Source: three-view drawing plus pictorial views. Frame: mm from the lowest corner of the part. A direction names the side the tool comes from. Give positions to 0.01 mm unless a question says otherwise; leave off trailing zeros. Loops run counter-clockwise (first coordinate to the right, second up) from the corner with the lowest first, then second, coordinate; pieces in that order, holes last. Notation, with made-up numbers: (78.25, -18.75) - (82.25, -18.75) arc R32 ccw to (82.25, 19.25) - close; hole circle Ø6 at (-17.75, -7.5). An arc over 180 degrees is marked (long way). One line per item, written item: value.
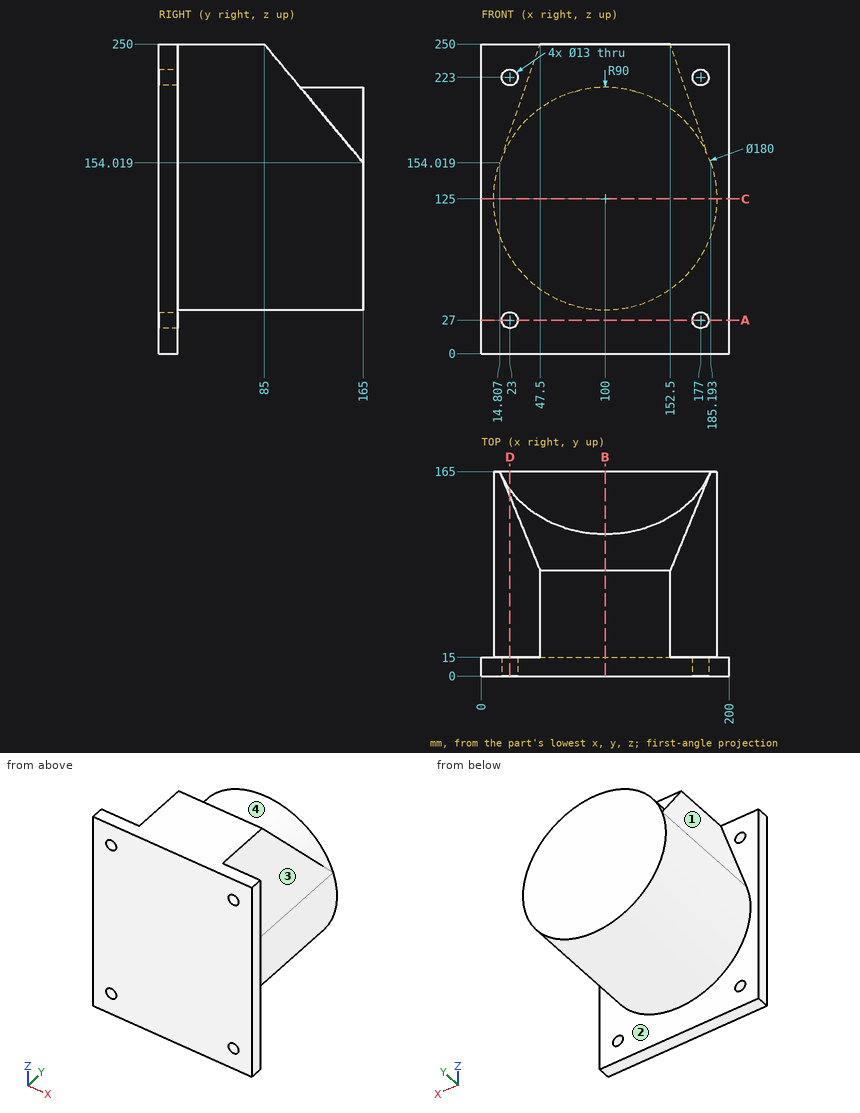
Item 1: Pin query (flat end, axial travel): P1, Ø3, axis at y = 24, z = 124, coming from the -X side; P2, Ø1, axis at y = 131.5, z = 206, coming from the +X side (1 decimal); P3, Ø2, axis at x = 113.5, y = 42, coming from the -Z side. Return the tip coordinate at first contact, or that it passes through.
Verdict:
P1: stops at x = 10
P2: stops at x = 140.2
P3: stops at z = 35.87
Item 2: Section A-A, the plane z = 27. Output: boundary loops of the cut face in (x, y).
Verdict:
outline: (0, 0) - (16.5, 0) - (16.5, 15) - (0, 15) - close; (29.5, 0) - (170.5, 0) - (170.5, 15) - (29.5, 15) - close; (183.5, 0) - (200, 0) - (200, 15) - (183.5, 15) - close
Item 3: Material intervals for L1, parallel to X at y = 9, z = 223; L2, parallel to Y at x = 184, z = 222; L3, parallel to Z at x = 139.5, y = 20.5, sorted ascending.
Verdict:
L1: x = 0 to 16.5, 29.5 to 170.5, 183.5 to 200
L2: y = 0 to 15
L3: z = 44.13 to 250
Item 4: Access query for the marked faces 1, 2, 3 and 4. Directions: +Z, -Z, +X, -X, +Y, -Y. A direction counts if a zero-diameter tool reaches every point of the face in a straight line with its end or side. Return the directions, or none.
Verdict:
face 1: +Z, -X, +Y
face 2: +Y
face 3: +Z, +X, +Y
face 4: +Z, +Y
Item 5: Section C-C, the plane z = 125. Output: boundary loops of the cut face in (x, y).
Verdict:
outline: (0, 0) - (200, 0) - (200, 15) - (190, 15) - (190, 165) - (10, 165) - (10, 15) - (0, 15) - close
Item 6: Section B-B, the plane x = 100. Output: boundary loops of the cut face in (y, z), and give its area (3 significant figures).
Verdict:
outline: (0, 0) - (15, 0) - (15, 35) - (165, 35) - (165, 215) - (114.17, 215) - (85, 250) - (0, 250) - close
area: 33,700 mm^2
Item 7: Section D-D, the plane x = 23. Output: boundary loops of the cut face in (y, z), and give its area (3 significant figures).
Verdict:
outline: (0, 0) - (15, 0) - (15, 20.5) - (0, 20.5) - close; (0, 33.5) - (15, 33.5) - (15, 78.41) - (165, 78.41) - (165, 171.59) - (150.35, 171.59) - (144.95, 178.07) - (15, 178.07) - (15, 216.5) - (0, 216.5) - close; (0, 229.5) - (15, 229.5) - (15, 250) - (0, 250) - close
area: 18,200 mm^2
